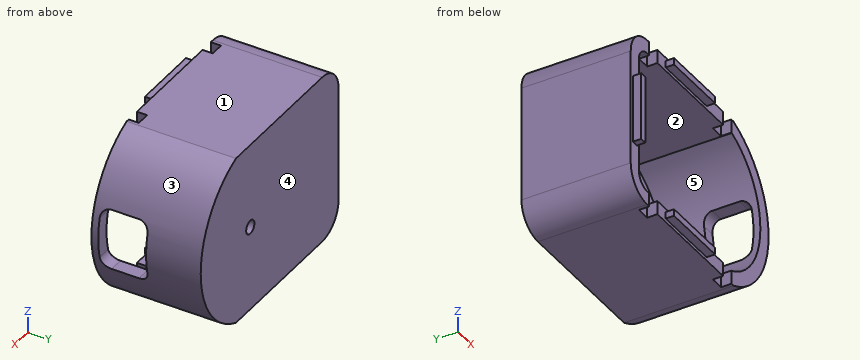
```python
from build123d import *

# Parameters (mm, degrees)
Y_KSEKLIK_EKSTR_ZYON1_DEPTH = 160
KES_EKSTR_ZYON1_DEPTH       = 140
IZIM3_W                     = 10
IZIM3_H                     = 100
IZIM3_W_2                   = 100
IZIM3_H_2                   = 10
Y_KSEKLIK_EKSTR_ZYON2_DEPTH = 12.3
IZIM4_R                     = 10
KES_EKSTR_ZYON2_DEPTH       = 641.3
KES_EKSTR_ZYON3_DEPTH       = 641.3
IZIM7_W                     = 20
IZIM7_H                     = 15
KES_EKSTR_ZYON4_DEPTH       = 641.3


with BuildPart() as part:
    # Çizim1 → Yükseklik-Ekstrüzyon1 (new body)
    with BuildSketch(Plane(origin=(0, 0, 0), x_dir=(1, 0, 0), z_dir=(0, 1, 0))):
        with BuildLine():
            Line((-127.864290172, 125), (82.135709828, 125))
            ThreePointArc((82.135709828, 125), (167.864290172, 0), (82.135709828, -125))
            Line((82.135709828, -125), (-127.864290172, -125))
            ThreePointArc((-127.864290172, -125), (-156.14856142, -113.284271247), (-167.864290172, -85))
            Line((-167.864290172, -85), (-167.864290172, 85))
            ThreePointArc((-167.864290172, 85), (-156.14856142, 113.284271247), (-127.864290172, 125))
        make_face()
    extrude(amount=-Y_KSEKLIK_EKSTR_ZYON1_DEPTH)

    # Çizim2 → Kes-Ekstrüzyon1 (cut)
    with BuildSketch(Plane.XZ.offset(160)):
        with BuildLine():
            Line((-127.864290172, -105), (78.252278635, -105))
            ThreePointArc((78.252278635, -105), (147.864290172, 0), (78.252278635, 105))
            Line((78.252278635, 105), (-127.864290172, 105))
            ThreePointArc((-127.864290172, 105), (-142.006425796, 99.142135624), (-147.864290172, 85))
            Line((-147.864290172, 85), (-147.864290172, -85))
            ThreePointArc((-147.864290172, -85), (-142.006425796, -99.142135624), (-127.864290172, -105))
        make_face()
    extrude(amount=-KES_EKSTR_ZYON1_DEPTH, mode=Mode.SUBTRACT)

    # Çizim3 → Yükseklik-Ekstrüzyon2 (add)
    with BuildSketch(Plane(origin=(0, -160, 0), x_dir=(-1, 0, 0), z_dir=(0, -1, 0))):
        with Locations((157.864290172, 0)):
            Rectangle(IZIM3_W, IZIM3_H)
        with Locations((32.864290172, 115)):
            Rectangle(IZIM3_W_2, IZIM3_H_2)
        with Locations((32.864290172, -115)):
            Rectangle(IZIM3_W_2, IZIM3_H_2)
    extrude(amount=Y_KSEKLIK_EKSTR_ZYON2_DEPTH)

    # Çizim4 → Kes-Ekstrüzyon2 (cut)
    with BuildSketch(Plane(origin=(0, 0, 0), x_dir=(1, 0, 0), z_dir=(0, 1, 0))):
        with Locations(Location((47.135709828, 0, 0), (0, 0, 270))):
            Circle(IZIM4_R)
    extrude(amount=-KES_EKSTR_ZYON2_DEPTH, mode=Mode.SUBTRACT)

    # Çizim6 → Kes-Ekstrüzyon3 (cut)
    with BuildSketch(Plane.ZY.offset(-62.135709828)):
        with BuildLine():
            Line((-30, -80), (30, -80))
            ThreePointArc((30, -80), (40.606601718, -84.393398282), (45, -95))
            Line((45, -95), (45, -135))
            ThreePointArc((45, -135), (40.606601718, -145.606601718), (30, -150))
            Line((30, -150), (-30, -150))
            ThreePointArc((-30, -150), (-40.606601718, -145.606601718), (-45, -135))
            Line((-45, -135), (-45, -95))
            ThreePointArc((-45, -95), (-40.606601718, -84.393398282), (-30, -80))
        make_face()
    extrude(amount=-KES_EKSTR_ZYON3_DEPTH, mode=Mode.SUBTRACT)

    # Çizim7 → Kes-Ekstrüzyon4 (cut)
    with BuildSketch(Plane.XY.offset(125)):
        with Locations((-112.864290172, -152.5)):
            Rectangle(IZIM7_W, IZIM7_H)
        with Locations((67.135709828, -152.5)):
            Rectangle(IZIM7_W, IZIM7_H)
    extrude(amount=-KES_EKSTR_ZYON4_DEPTH, mode=Mode.SUBTRACT)


solid = part.part
```
Can you work these out from the model? Positions are in its coordinate system, mm. Face numbers are marked on the shaded views. A direction names the side the tool comes from. Coordinates: 2 decimals unless noted, no trailing zeros. Loops run counter-clockwise (first coordinate to the right, second up) from the corner with the lowest first, then second, coordinate; pieces in that order, holes last. Notation, with made-up numbers: (-22.5, 55.25) - (-10.5, 55.25) arc R34 ccw to (-10.5, 92.25) - close; hole circle Ø11 at (60, 40.5). An arc over 180 degrees is marked (long way). Use a Markdown table: item, result.
Item 1: I want a section at D-D on x = -9.5. Please give me the cut outline in (y, z), and give its area (3 significant figures).
Numbers:
| item | result |
|---|---|
| outline | (-172.3, -120) - (-160, -120) - (-160, -125) - (0, -125) - (0, 125) - (-160, 125) - (-160, 120) - (-172.3, 120) - (-172.3, 110) - (-160, 110) - (-160, 105) - (-20, 105) - (-20, -105) - (-160, -105) - (-160, -110) - (-172.3, -110) - close |
| area | 10,800 mm2 |
Item 2: Will these pins go through, and if not, where does the flat tip stop? pin 1 (10 mm diameter, centred on x = -111.5, z = -120, fed in from -Y); pin 2 (5 mm diameter, centred on y = -168, z = -114.5, fed in from +X); pin 3 (7.5 mm diameter, centred on y = -152.5, z = -118.5, fed in from +X); pin 4 (3 mm diameter, centred on x = 12.5, z = 57, fed in from +Y).
Numbers:
| item | result |
|---|---|
| pin 1 | stops at y = -145 |
| pin 2 | stops at x = 17.14 |
| pin 3 | stops at x = 103.06 |
| pin 4 | stops at y = 0 |
Item 3: I want a section at A-A on z = 0. Please give me the cut outline in (x, y), and give its area (3 significant figures).
Numbers:
| item | result |
|---|---|
| outline | (-167.86, -160) - (-162.86, -160) - (-162.86, -172.3) - (-152.86, -172.3) - (-152.86, -160) - (-147.86, -160) - (-147.86, -20) - (37.14, -20) - (37.14, 0) - (-167.86, 0) - close; (57.14, -20) - (147.86, -20) - (147.86, -80) - (167.86, -80) - (167.86, 0) - (57.14, 0) - close; (147.86, -160) - (167.86, -160) - (167.86, -150) - (147.86, -150) - close |
| area | 10,600 mm2 |
Item 4: If I drill on probe 1 along Z at (x, y) = (-122, -141); probe 2 along X at (y, z) = (-10, 0); probe 3 along Y at (x, z) = (125, 96), over which ranges is the centre line in solid material (lowest first)? Write a range as from..to.
Numbers:
| item | result |
|---|---|
| probe 1 | z = -125..-105, 105..125 |
| probe 2 | x = -167.86..37.14, 57.14..167.86 |
| probe 3 | y = -160..0 |
Item 5: I want a section at B-B on y = -155. Please give me the cut outline in (x, z).
Numbers:
| item | result |
|---|---|
| outline | (-167.86, -85) arc R40 ccw to (-127.86, -125) - (-122.86, -125) - (-122.86, -105) - (-127.86, -105) arc R20 cw to (-147.86, -85) - (-147.86, 85) arc R20 cw to (-127.86, 105) - (-122.86, 105) - (-122.86, 125) - (-127.86, 125) arc R40 ccw to (-167.86, 85) - close; (-102.86, -125) - (57.14, -125) - (57.14, -105) - (-102.86, -105) - close; (-102.86, 105) - (57.14, 105) - (57.14, 125) - (-102.86, 125) - close; (77.14, -125) - (82.14, -125) arc R133.99 ccw to (82.14, 125) - (77.14, 125) - (77.14, 105) - (78.25, 105) arc R113.99 cw to (78.25, -105) - (77.14, -105) - close |
Item 6: For the marked faces 4 and 5, which set-ups out of +Z, -Z, +X, -X, +Y, -Y let a thin tool reach every point of the face, with its end or its side?
Numbers:
| item | result |
|---|---|
| face 4 | +Z, -Z, +X, -X, +Y |
| face 5 | -Y |
Item 7: We'd pull the mould along Z, two halves only. Please class the marked faces 1, 2 and 3: released by +Z, released by -Z, zero draft, split by the parting line, or undercut.
Numbers:
| item | result |
|---|---|
| face 1 | released by +Z |
| face 2 | undercut |
| face 3 | split by the parting line |
Item 8: I want a section at C-C on y = -115.5. Please give me the cut outline in (x, z), and give its area (3 significant figures).
Numbers:
| item | result |
|---|---|
| outline | (-167.86, -85) arc R40 ccw to (-127.86, -125) - (82.14, -125) arc R133.99 ccw to (160.08, -45) - (138.61, -45) arc R113.99 cw to (78.25, -105) - (-127.86, -105) arc R20 cw to (-147.86, -85) - (-147.86, 85) arc R20 cw to (-127.86, 105) - (78.25, 105) arc R113.99 cw to (138.61, 45) - (160.08, 45) arc R133.99 ccw to (82.14, 125) - (-127.86, 125) arc R40 ccw to (-167.86, 85) - close |
| area | 17,700 mm2 |
